```python
from build123d import *

# Parameters (mm, degrees)
SKETCH1_W                   = 50
SKETCH1_H                   = 106.4
BOSS_EXTRUDE1_DEPTH         = 5
SKETCH2_W                   = 20
SKETCH2_H                   = 3
BOSS_EXTRUDE2_DEPTH         = 4
TAP_DRILL_FOR_M2X0_4_TAP1_D = 2.2
LPATTERN1_COUNT             = 4
LPATTERN1_PITCH             = 15
LPATTERN1_COL_COUNT         = 4
LPATTERN1_COL_PITCH         = 15
CUT_EXTRUDE1_DEPTH          = 118.668857392
SKETCH7_W                   = 11.1694
SKETCH7_H                   = 71.9308
CUT_EXTRUDE2_DEPTH          = 3
F_2_CLEARANCE_HOLE1_D       = 2.7051
SKETCH11_R                  = 1.8
CUT_EXTRUDE3_DEPTH          = 118.906573184
BOSS_EXTRUDE5_DEPTH         = 6.731
BOSS_EXTRUDE5_DEPTH_BACK    = 56.769
SKETCH14_W                  = 7.277473249
SKETCH14_H                  = 8.107504071
SKETCH14_R                  = 2.54
SKETCH14_W_2                = 8.508813203
SKETCH14_H_2                = 9.759110034
SKETCH15_W                  = 3.3655
SKETCH15_H                  = 8.107504071
SKETCH15_W_2                = 3.3845
BOSS_EXTRUDE6_DEPTH         = 4.731
CUT_EXTRUDE4_REACH          = 123.844
SKETCH16_W                  = 43.18
SKETCH16_H                  = 8.107504071
SKETCH16_W_2                = 21.67
SKETCH16_H_2                = 9.759110034


with BuildPart() as part:
    # Sketch1 → Boss-Extrude1 (new body)
    with BuildSketch(Plane.XY):
        with Locations((25, 53.2)):
            Rectangle(SKETCH1_W, SKETCH1_H)
    extrude(amount=BOSS_EXTRUDE1_DEPTH)

    # Sketch2 → Boss-Extrude2 (add)
    with BuildSketch(Plane.XY.offset(5)):
        with Locations((25, 104.9)):
            Rectangle(SKETCH2_W, SKETCH2_H)
    boss_extrude2 = extrude(amount=BOSS_EXTRUDE2_DEPTH)

    # Mirror1: Boss-Extrude2 across plane
    add(boss_extrude2.mirror(Plane.ZX.offset(53.2)))

    # Tap Drill for M2x0.4 Tap1 (through all)
    with Locations(Plane.XY.offset(5)):
        with Locations((25, 53.2)):
            tap_drill_for_m2x0_4_tap1 = Hole(TAP_DRILL_FOR_M2X0_4_TAP1_D / 2)

    # LPattern1: Tap Drill for M2x0.4 Tap1 ×4
    with Locations(*[(0, -i * LPATTERN1_PITCH, 0) for i in range(1, LPATTERN1_COUNT)]):
        add(tap_drill_for_m2x0_4_tap1, mode=Mode.SUBTRACT)

    # LPattern1 col: Tap Drill for M2x0.4 Tap1 ×4
    with Locations(*[(0, i * LPATTERN1_COL_PITCH, 0) for i in range(1, LPATTERN1_COL_COUNT)]):
        add(tap_drill_for_m2x0_4_tap1, mode=Mode.SUBTRACT)

    # Sketch6 → Cut-Extrude1 (cut, through all)
    with BuildSketch(Plane.XY.offset(5)):
        with BuildLine():
            Line((11.2347, 7.1336), (11.2347, 73.0644))
            ThreePointArc((11.2347, 73.0644), (12.5847, 74.4144), (13.9347, 73.0644))
            Line((13.9347, 73.0644), (13.9347, 7.1336))
            ThreePointArc((13.9347, 7.1336), (12.5847, 5.7836), (11.2347, 7.1336))
        make_face()
    extrude(amount=-CUT_EXTRUDE1_DEPTH, mode=Mode.SUBTRACT)

    # Sketch7 → Cut-Extrude2 (cut)
    with BuildSketch(Plane(origin=(0, 0, 0), x_dir=(-1, 0, 0), z_dir=(0, 0, -1))):
        with Locations((-12.5847, 40.099)):
            Rectangle(SKETCH7_W, SKETCH7_H)
    extrude(amount=-CUT_EXTRUDE2_DEPTH, mode=Mode.SUBTRACT)

    # #2 Clearance Hole1 (through all)
    with Locations(Plane(origin=(0, 0, 0), x_dir=(-1, 0, 0), z_dir=(0, 0, -1))):
        with Locations((-47.5, 45.3), (-2.5, 45.3), (-2.5, 15), (-47.5, 15)):
            Hole(F_2_CLEARANCE_HOLE1_D / 2)

    # Sketch11 → Cut-Extrude3 (cut, through all)
    with BuildSketch(Plane(origin=(0, 0, 0), x_dir=(-1, 0, 0), z_dir=(0, 0, -1))):
        with BuildLine():
            Line((-46.795, 98.2156), (-46.795, 95.7156))
            ThreePointArc((-46.795, 95.7156), (-44.995, 97.5156), (-43.195, 95.7156))
            Line((-43.195, 95.7156), (-43.195, 98.2156))
            ThreePointArc((-43.195, 98.2156), (-44.995, 100.0156), (-46.795, 98.2156))
        make_face()
        with Locations((-44.995, 95.7156)):
            Circle(SKETCH11_R)
        with BuildLine():
            Line((-46.795, 95.7156), (-46.795, 93.2156))
            ThreePointArc((-46.795, 93.2156), (-44.995, 91.4156), (-43.195, 93.2156))
            Line((-43.195, 93.2156), (-43.195, 95.7156))
            ThreePointArc((-43.195, 95.7156), (-44.995, 93.9156), (-46.795, 95.7156))
        make_face()
        with BuildLine():
            Line((-6.795, 98.2156), (-6.795, 95.715599993))
            ThreePointArc((-6.795, 95.715599993), (-4.995000003, 97.5156), (-3.195, 95.7156))
            Line((-3.195, 95.7156), (-3.195, 98.2156))
            ThreePointArc((-3.195, 98.2156), (-4.995, 100.0156), (-6.795, 98.2156))
        make_face()
        with Locations((-4.995, 95.7156)):
            Circle(SKETCH11_R)
        with BuildLine():
            Line((-6.795, 95.715599993), (-6.795, 93.2156))
            ThreePointArc((-6.795, 93.2156), (-4.995, 91.4156), (-3.195, 93.2156))
            Line((-3.195, 93.2156), (-3.195, 95.7156))
            ThreePointArc((-3.195, 95.7156), (-4.994999997, 93.9156), (-6.795, 95.715599993))
        make_face()
    extrude(amount=-CUT_EXTRUDE3_DEPTH, mode=Mode.SUBTRACT)

    # Sketch14 → Boss-Extrude5 (add, two sides: drawn at the far end of the back side and taken through both)
    # profile 1 of 2: a face of its own
    with BuildSketch(Plane(origin=(50, 0, 0), x_dir=(0, 0, -1), z_dir=(1, 0, 0)).offset(-BOSS_EXTRUDE5_DEPTH_BACK)):
        with Locations((3.638736625, 21.708366631)):
            Rectangle(SKETCH14_W, SKETCH14_H)
        with Locations((2.980230777, 22)):
            Circle(SKETCH14_R, mode=Mode.SUBTRACT)
    # profile 2 of 2: a face of its own
    with BuildSketch(Plane(origin=(50, 0, 0), x_dir=(0, 0, -1), z_dir=(1, 0, 0)).offset(-BOSS_EXTRUDE5_DEPTH_BACK)):
        with Locations((4.254406602, 85.657429776)):
            Rectangle(SKETCH14_W_2, SKETCH14_H_2)
        with Locations((2.980230777, 85.5)):
            Circle(SKETCH14_R, mode=Mode.SUBTRACT)
    extrude(amount=BOSS_EXTRUDE5_DEPTH + BOSS_EXTRUDE5_DEPTH_BACK)

    # Sketch15 → Boss-Extrude6 (add)
    with BuildSketch(Plane.XY):
        with Locations((51.68275, 21.708366631)):
            Rectangle(SKETCH15_W, SKETCH15_H)
        with Locations((-1.69225, 21.708366631)):
            Rectangle(SKETCH15_W_2, SKETCH15_H)
    extrude(amount=BOSS_EXTRUDE6_DEPTH)

    # Cut-Extrude4: up to this face of the body (flat: up to its plane)
    cut_extrude4_end = Plane(part.part.faces().sort_by_distance((28.220383902, 53.923969289, 0))[0])
    # Sketch16 → Cut-Extrude4 (cut, up to the picked face)
    with BuildSketch(Plane(origin=(0, 0, -8.508813203), x_dir=(-1, 0, 0), z_dir=(0, 0, -1)), mode=Mode.PRIVATE) as cut_extrude4_sk1:
        with Locations((-24.981, 21.708366631)):
            Rectangle(SKETCH16_W, SKETCH16_H)
    cut_extrude4_tool1 = split(extrude(cut_extrude4_sk1.sketch, amount=-CUT_EXTRUDE4_REACH, mode=Mode.PRIVATE), bisect_by=cut_extrude4_end, keep=Keep.BOTH, mode=Mode.PRIVATE)
    # Sketch16 → Cut-Extrude4 (cut, up to the picked face)
    with BuildSketch(Plane(origin=(0, 0, -8.508813203), x_dir=(-1, 0, 0), z_dir=(0, 0, -1)), mode=Mode.PRIVATE) as cut_extrude4_sk2:
        Polygon((-19.901, 80.777874759), (-30.061, 90.536984793), (-30.061, 80.777874759), align=None)
    cut_extrude4_tool2 = split(extrude(cut_extrude4_sk2.sketch, amount=-CUT_EXTRUDE4_REACH, mode=Mode.PRIVATE), bisect_by=cut_extrude4_end, keep=Keep.BOTH, mode=Mode.PRIVATE)
    # Sketch16 → Cut-Extrude4 (cut, up to the picked face)
    with BuildSketch(Plane(origin=(0, 0, -8.508813203), x_dir=(-1, 0, 0), z_dir=(0, 0, -1)), mode=Mode.PRIVATE) as cut_extrude4_sk3:
        Polygon((-19.901, 90.536984793), (-30.061, 90.536984793), (-19.901, 80.777874759), align=None)
    cut_extrude4_tool3 = split(extrude(cut_extrude4_sk3.sketch, amount=-CUT_EXTRUDE4_REACH, mode=Mode.PRIVATE), bisect_by=cut_extrude4_end, keep=Keep.BOTH, mode=Mode.PRIVATE)
    # Sketch16 → Cut-Extrude4 (cut, up to the picked face)
    with BuildSketch(Plane(origin=(0, 0, -8.508813203), x_dir=(-1, 0, 0), z_dir=(0, 0, -1)), mode=Mode.PRIVATE) as cut_extrude4_sk4:
        with Locations((-45.896, 85.657429776)):
            Rectangle(SKETCH16_W_2, SKETCH16_H_2)
    cut_extrude4_tool4 = split(extrude(cut_extrude4_sk4.sketch, amount=-CUT_EXTRUDE4_REACH, mode=Mode.PRIVATE), bisect_by=cut_extrude4_end, keep=Keep.BOTH, mode=Mode.PRIVATE)
    # Sketch16 → Cut-Extrude4 (cut, up to the picked face)
    with BuildSketch(Plane(origin=(0, 0, -8.508813203), x_dir=(-1, 0, 0), z_dir=(0, 0, -1)), mode=Mode.PRIVATE) as cut_extrude4_sk5:
        with Locations((-4.066, 85.657429776)):
            Rectangle(SKETCH16_W_2, SKETCH16_H_2)
    cut_extrude4_tool5 = split(extrude(cut_extrude4_sk5.sketch, amount=-CUT_EXTRUDE4_REACH, mode=Mode.PRIVATE), bisect_by=cut_extrude4_end, keep=Keep.BOTH, mode=Mode.PRIVATE)
    add(cut_extrude4_tool1.solids().sort_by(Axis((24.981, 21.708367, -8.508813), (0, 0, 1)))[0], mode=Mode.SUBTRACT)
    add(cut_extrude4_tool2.solids().sort_by(Axis((26.674333, 84.030911, -8.508813), (0, 0, 1)))[0], mode=Mode.SUBTRACT)
    add(cut_extrude4_tool3.solids().sort_by(Axis((23.287667, 87.283948, -8.508813), (0, 0, 1)))[0], mode=Mode.SUBTRACT)
    add(cut_extrude4_tool4.solids().sort_by(Axis((45.896, 85.65743, -8.508813), (0, 0, 1)))[0], mode=Mode.SUBTRACT)
    add(cut_extrude4_tool5.solids().sort_by(Axis((4.066, 85.65743, -8.508813), (0, 0, 1)))[0], mode=Mode.SUBTRACT)


solid = part.part
```
Build history of the part. All positions in model axes, mm. A direction names the side the tool comes from. Coordinates: 2 decimals unless noted, no trailing zeros. Order: outer loops, then holes, each group sorted by start corner. A loop starts at its lowest first (then second) coordinate and runs counter-clockwise, first axis right, second up. Notation, with made-up numbers: (-38.5, -30) -> (14.5, -30) arc R10 ccw to (14.5, -17) -> close; hole circle Ø10 at (8.5, 83). An arc over 180 degrees is marked (long way). Answer in a Markdown table with one row per item. Add a question column.
Q1. Drop flat-ended pins along their axis: pin 1 (2.5 mm diameter, centred on y = 20, z = 3, fed in from -X); pin 2 (3.5 mm diameter, centred on y = 28.5, z = 1.5, fed in from -X); pin 3 (2.5 mm diameter, centred on y = 1, z = 7, fed in from -X); pin 4 (1.8 mm diameter, centred on x = 25, y = 8.2, fed in from +Z). Give the stop position or say it passes through.
Q2. Band-saw the part on D-D, the plane y = 85.5. List the corners of the cut face in (x, z).
Q3. Band-saw the part on B-B, the plane y = 45.3. List the corners of the cut face in (x, z).
Q4. Wall check: line 1 along Y through (x, z) = (29, 6.5); line 2 along Z through (x, y) = (54.5, 22); line 3 along X through (y, z) = (55, 1.5). Give the ranges that are in metal, low to high. Write a range as [from, to].
Q5. Band-saw the part on C-C, the plane x = 45. List the corners of the cut face in (y, z), then the cut area to 3 significant figures.
Q6. Mould opens along X. For faces 1 (the face through (15, 105, 7)), 2 (the face through (30, 54, 5)), 3 (the face through (3.195, 96, 2)) say: +X half, -X half, draft (parallel to the pull), parting line (faces both ways), or undercut.
Q7. Which spindle directions (+Z, -Z, +X, -X, +Y, -Y) get a long thin tool onto all of the face, cutting with end or side? Do faces 4 (the face through (55, 22, 0)), 5 (the face through (17, 90.537, -4)), 6 (the face through (10, 41, 3)), 7 (the face through (13.935, 41, 4)), 8 (the face through (-3.384, 22, 2)). Say none if no direction does.
Q8. Band-saw the part on A-A, the plane y = 32. List the corners of the cut face in (x, z).
Answers follow:
| question | item | result |
|---|---|---|
| 1 | pin 1 | x = -3.38 |
| 1 | pin 2 | x = 0 |
| 1 | pin 3 | x = 15 |
| 1 | pin 4 | through |
| 2 | outline | (0, 0) -> (14.9, 0) -> (14.9, -0.44) -> (19.9, -0.44) -> (19.9, 0) -> (30.06, 0) -> (30.06, -0.44) -> (35.06, -0.44) -> (35.06, 0) -> (50, 0) -> (50, 5) -> (0, 5) -> close; (14.9, -8.51) -> (19.9, -8.51) -> (19.9, -5.52) -> (14.9, -5.52) -> close; (30.06, -8.51) -> (35.06, -8.51) -> (35.06, -5.52) -> (30.06, -5.52) -> close |
| 3 | outline | (0, 0) -> (1.15, 0) -> (1.15, 5) -> (0, 5) -> close; (3.85, 0) -> (7, 0) -> (7, 3) -> (11.23, 3) -> (11.23, 5) -> (3.85, 5) -> close; (13.93, 3) -> (18.17, 3) -> (18.17, 0) -> (46.15, 0) -> (46.15, 5) -> (13.93, 5) -> close; (48.85, 0) -> (50, 0) -> (50, 5) -> (48.85, 5) -> close |
| 4 | line 1 | [0, 3], [103.4, 106.4] |
| 4 | line 2 | [-7.28, -5.52], [-0.44, 0] |
| 4 | line 3 | [0, 7], [18.17, 50] |
| 5 | outline | (0, 0) -> (91.42, 0) -> (91.42, 5) -> (0, 5) -> close; (100.02, 0) -> (106.4, 0) -> (106.4, 5) -> (100.02, 5) -> close |
| 5 | area | 489 mm^2 |
| 6 | face 1 | -X half |
| 6 | face 2 | draft |
| 6 | face 3 | undercut |
| 7 | face 4 | +Z, +X, +Y, -Y |
| 7 | face 5 | -Z, +X, -X, +Y |
| 7 | face 6 | -Z |
| 7 | face 7 | +Z, -Z |
| 7 | face 8 | +Z, -X, +Y, -Y |
| 8 | outline | (0, 0) -> (7, 0) -> (7, 3) -> (11.23, 3) -> (11.23, 5) -> (0, 5) -> close; (13.93, 3) -> (18.17, 3) -> (18.17, 0) -> (50, 0) -> (50, 5) -> (13.93, 5) -> close |
